Check sheet for the modelled part. Datum: model origin and axes. Units: mm. Round coordinates to 2 decimals unless told otherwise and drop trailing zeros. Order: outer loops, then holes, each group sorted by start corner. A loop starts at its lowest first (then second) coordinate and runs counter-clockwise, first axis right, second up.
Q1. Cross-section at A-A on y = 5. Record the cut outline in (x, z), then the cut area to 3 significant figures.
Q2. Cross-section at D-D on z = 2.2. Give the number of separate pieces and of enclosed holes in the cut face, then the cut area to 3 significant figures.
Q3. Cross-section at B-B on x = 10. Record the cut outline in (y, z).
Q4. Scan lines: probe 1 along Y at (x, z) = (62.5, 1.3); probe 2 along X at (y, z) = (89.5, 0.25); probe 3 along X at (y, z) = (33, 0.6). Record each from-to range of solid material in increasing order.
Q5. Cross-section at C-C on x = 72.5. Record the cut outline in (y, z).
Q6. Depth check by flat-ended pin: P1, Ø12, axis at x = 28.5, y = 93.5, coming from the -Z side. Enter the tip coordinate at first touch or a pass-through.
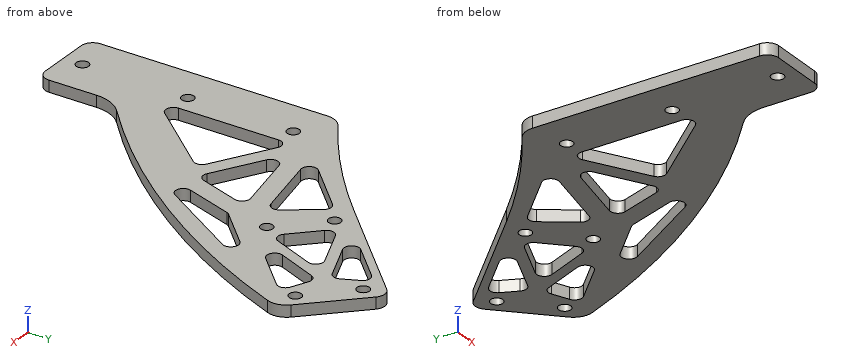
from build123d import *

# Parameters (mm, degrees)
SKETCH_1_W          = 20
SKETCH_1_H          = 65
EXTRUDE_1_DEPTH     = 3
SKETCH_2_R          = 1.6
CUT_EXTRUDE_1_DEPTH = 3
EXTRUDE_2_DEPTH     = 3
EXTRUDE_3_DEPTH     = 3
SKETCH_8_R          = 1.6
CUT_EXTRUDE_3_DEPTH = 143.659058168
FILLET_1_R          = 10
FILLET_2_R          = 3
FILLET_3_R          = 5
CUT_EXTRUDE_4_DEPTH = 142.149179722
FILLET_4_R          = 2


with BuildPart() as part:
    # Sketch 1 → Extrude 1 (new body)
    with BuildSketch(Plane.XY):
        with Locations((10, 32.5)):
            Rectangle(SKETCH_1_W, SKETCH_1_H)
    extrude(amount=EXTRUDE_1_DEPTH)

    # Sketch 2 → Cut-Extrude 1 (cut)
    with BuildSketch(Plane.XY.offset(3)):
        with Locations((10, 60)):
            Circle(SKETCH_2_R)
        with Locations((10, 32.5)):
            Circle(SKETCH_2_R)
        with Locations((10, 5)):
            Circle(SKETCH_2_R)
    extrude(amount=-CUT_EXTRUDE_1_DEPTH, mode=Mode.SUBTRACT)



with BuildPart() as body_2:
    # Sketch 3 → Extrude 2 (new body)
    with BuildSketch(Plane.XY.offset(3)):
        Polygon((32.478445072, 90.836309448), (50.156114601, 73.158639918), (78.440385849, 101.442911166), (60.762716319, 119.120580695), align=None)
    extrude(amount=-EXTRUDE_2_DEPTH)


with BuildPart() as part_1:
    add(part.part)

    add(body_2.part)  # Extrude 3 merges body 2
    # Sketch 4 → Extrude 3 (add)
    with BuildSketch(Plane.XY.offset(3)):
        with BuildLine():
            Line((78.440385849, 101.442911166), (50.156114601, 73.158639918))
            Line((50.156114601, 73.158639918), (32.478445072, 90.836309448))
            ThreePointArc((32.478445072, 90.836309448), (16.972550072, 76.996299451), (0, 65))
            Line((0, 65), (20, 65))
            Line((20, 65), (20, 20))
            ThreePointArc((20, 20), (54.405363127, 57.00077145), (78.440385849, 101.442911166))
        make_face()
    extrude(amount=-EXTRUDE_3_DEPTH)

    # Sketch 8 → Cut-Extrude 3 (cut, through all)
    with BuildSketch(Plane.XY.offset(3)):
        with Locations((61.4698231, 112.756619665)):
            Circle(SKETCH_8_R)
        with Locations((72.076424818, 102.150017947)):
            Circle(SKETCH_8_R)
        with Locations((49.44900782, 79.522600949)):
            Circle(SKETCH_8_R)
        with Locations((38.842406102, 90.129202667)):
            Circle(SKETCH_8_R)
    extrude(amount=-CUT_EXTRUDE_3_DEPTH, mode=Mode.SUBTRACT)

    # Fillet 1
    fillet_1_edges = [part_1.edges().sort_by_distance(p)[0] for p in [
        (20, 20, 1.5),
    ]]
    fillet(fillet_1_edges, radius=FILLET_1_R)

    # Fillet 2
    fillet_2_edges = [part_1.edges().sort_by_distance(p)[0] for p in [
        (60.762716319, 119.120580695, 1.5),
        (20, 0, 1.5),
        (0, 0, 1.5),
    ]]
    fillet(fillet_2_edges, radius=FILLET_2_R)

    # Fillet 3
    fillet_3_edges = [part_1.edges().sort_by_distance(p)[0] for p in [
        (78.440385849, 101.442911166, 1.5),
        (0, 65, 1.5),
    ]]
    fillet(fillet_3_edges, radius=FILLET_3_R)

    # Sketch 10 → Cut-Extrude 4 (cut, through all)
    with BuildSketch(Plane.XY.offset(3)):
        Polygon((16.922095886, 69.623106012), (34.599765415, 87.300775542), (43.20341196, 75.013494878), align=None)
        Polygon((19.465452368, 65.040672027), (43.955639167, 70.06369408), (38.60577187, 53.99000341), align=None)
        Polygon((15, 63), (35, 51.452994616), (15, 28), align=None)
        Polygon((39.549512883, 95.078950135), (57.227182413, 112.756619665), (61.186980388, 103.988495578), align=None)
        Polygon((41.670833227, 92.957629791), (59.702056147, 100.382250994), (52.277434945, 82.351028074), align=None)
        Polygon((63.308300731, 101.867175234), (54.398755288, 80.22970773), (72.076424818, 97.90737726), align=None)
        Polygon((48.893917057, 69.06801525), (39.281396308, 40.187170828), (70.417203629, 90.591301821), align=None)
    extrude(amount=-CUT_EXTRUDE_4_DEPTH, mode=Mode.SUBTRACT)

    # Fillet 4
    fillet_4_edges = [part_1.edges().sort_by_distance(p)[0] for p in [
        (15, 28, 1.5),
        (15, 63, 1.5),
        (35, 51.452994616, 1.5),
        (38.60577187, 53.99000341, 1.5),
        (19.465452368, 65.040672027, 1.5),
        (43.955639167, 70.06369408, 1.5),
        (52.277434945, 82.351028074, 1.5),
        (41.670833227, 92.957629791, 1.5),
        (59.702056147, 100.382250994, 1.5),
        (61.186980388, 103.988495578, 1.5),
        (39.549512883, 95.078950135, 1.5),
        (57.227182413, 112.756619665, 1.5),
        (48.893917057, 69.06801525, 1.5),
        (70.417203629, 90.591301821, 1.5),
        (39.281396308, 40.187170828, 1.5),
        (63.308300731, 101.867175234, 1.5),
        (72.076424818, 97.90737726, 1.5),
        (54.398755288, 80.22970773, 1.5),
        (43.20341196, 75.013494878, 1.5),
        (16.922095886, 69.623106012, 1.5),
        (34.599765415, 87.300775542, 1.5),
    ]]
    fillet(fillet_4_edges, radius=FILLET_4_R)


solid = part_1.part
Results found:
1. outline: (0, 0) - (8.4, 0) - (8.4, 3) - (0, 3) - close; (11.6, 0) - (20, 0) - (20, 3) - (11.6, 3) - close
1. area: 50.4 mm2
2. separate pieces: 1
2. enclosed holes: 14
2. area: 3,080 mm2
3. outline: (0, 0) - (3.4, 0) - (3.4, 3) - (0, 3) - close; (6.6, 0) - (30.9, 0) - (30.9, 3) - (6.6, 3) - close; (34.1, 0) - (58.4, 0) - (58.4, 3) - (34.1, 3) - close; (61.6, 0) - (71.72, 0) - (71.72, 3) - (61.6, 3) - close
4. probe 1: y = 69.2 to 88.33, 99.9 to 111.53, 113.98 to 117.32
4. probe 2: x = 31.13 to 37.37, 40.31 to 45.13, 55.22 to 58.22, 63.67 to 73.37
4. probe 3: x = 0 to 8.48, 11.52 to 15.05, 19.26 to 34.15
5. outline: (87.65, 0) - (100.61, 0) - (100.61, 3) - (87.65, 3) - close; (103.69, 0) - (107.38, 0) - (107.38, 3) - (103.69, 3) - close
6. P1: stops at z = 0
